Geometry: final body of the model. Coordinates: model frame, mm. A direction names the side the tool comes from. Give positions to 0.01 mm unless a question says otherwise; leave off trailing zeros. Loops run counter-clockwise (first coordinate to the right, second up) from the corner with the lowest first, then second, coordinate; pieces in that order, holes last. Notation, with made-up numbers: (-22.5, -3) - (19.5, -3) arc R19 cw to (19.5, 22) - close; hole circle Ø4 at (29, 15.25). An arc over 180 degrees is marked (long way). Answer in a Markdown table with one row per item.
from build123d import *

# Parameters (mm, degrees)
SKETCH1_W           = 37.338
SKETCH1_H           = 38.1
BOSS_EXTRUDE1_DEPTH = 63.5
SKETCH3_W           = 37.338
SKETCH3_H           = 10.16
CUT_EXTRUDE1_DEPTH  = 38.1
SKETCH4_W           = 37.338
SKETCH4_H           = 17.145
CUT_EXTRUDE2_DEPTH  = 19.05
SKETCH5_W           = 33.782
SKETCH5_H           = 10.16
CUT_EXTRUDE3_DEPTH  = 47.508537507
SKETCH6_W           = 2.54
SKETCH6_H           = 38.1
SKETCH6_W_2         = 1.778
CUT_EXTRUDE4_DEPTH  = 31.75


with BuildPart() as part:
    # Sketch1 → Boss-Extrude1 (new body)
    with BuildSketch(Plane(origin=(0, 0, 0), x_dir=(1, 0, 0), z_dir=(0, 1, 0))):
        Rectangle(SKETCH1_W, SKETCH1_H)
    extrude(amount=BOSS_EXTRUDE1_DEPTH)

    # Sketch3 → Cut-Extrude1 (cut)
    with BuildSketch(Plane(origin=(0, 63.5, 0), x_dir=(1, 0, 0), z_dir=(0, 1, 0))):
        Rectangle(SKETCH3_W, SKETCH3_H)
    extrude(amount=-CUT_EXTRUDE1_DEPTH, mode=Mode.SUBTRACT)

    # Sketch4 → Cut-Extrude2 (cut)
    with BuildSketch(Plane.XZ):
        Rectangle(SKETCH4_W, SKETCH4_H)
    extrude(amount=-CUT_EXTRUDE2_DEPTH, mode=Mode.SUBTRACT)

    # Sketch5 → Cut-Extrude3 (cut, through all)
    with BuildSketch(Plane(origin=(0, 25.4, 0), x_dir=(1, 0, 0), z_dir=(0, 1, 0))):
        Rectangle(SKETCH5_W, SKETCH5_H)
    extrude(amount=-CUT_EXTRUDE3_DEPTH, mode=Mode.SUBTRACT)

    # Sketch6 → Cut-Extrude4 (cut)
    with BuildSketch(Plane(origin=(0, 63.5, 0), x_dir=(1, 0, 0), z_dir=(0, 1, 0))):
        with Locations((17.399, 0)):
            Rectangle(SKETCH6_W, SKETCH6_H)
        with Locations((-17.78, 0)):
            Rectangle(SKETCH6_W_2, SKETCH6_H)
    extrude(amount=-CUT_EXTRUDE4_DEPTH, mode=Mode.SUBTRACT)


solid = part.part
Q1. Cut plane A-A (z = -1.5). Output: boundary loops of the cut face in (x, y), and give its area (3 significant figures).
Check values:
| item | result |
|---|---|
| outline | (-18.67, 19.05) - (-16.89, 19.05) - (-16.89, 25.4) - (-18.67, 25.4) - close; (16.89, 19.05) - (18.67, 19.05) - (18.67, 25.4) - (16.89, 25.4) - close |
| area | 22.6 mm² |
Q2. Material intervals for line 1 along Z through (x, y) = (5.5, 7.5); line 2 along Z through (x, y) = (-3.5, 43.5); line 3 along X through (y, z) = (52.5, 15), sorted ascending.
Check values:
| item | result |
|---|---|
| line 1 | -19.05 to -8.57, 8.57 to 19.05 |
| line 2 | -19.05 to -5.08, 5.08 to 19.05 |
| line 3 | -16.89 to 16.13 |
Q3. Cut plane D-D (z = 14). Output: boundary loops of the cut face in (x, y), and give its area (3 significant figures).
Check values:
| item | result |
|---|---|
| outline | (-18.67, 0) - (18.67, 0) - (18.67, 31.75) - (16.13, 31.75) - (16.13, 63.5) - (-16.89, 63.5) - (-16.89, 31.75) - (-18.67, 31.75) - close |
| area | 2,230 mm² |
Q4. Draft query along X for faces 1 (the flat face through (0, 42, -5.08)), 2 (the flat face through (18.669, 23, 0)), 3 (the flat face through (0, 9, -8.572)). Return one class per face: pulls with the +X half, pulls with the -X half, needs draft (parallel to the pull), parting line crosses it, or undercut.
Check values:
| item | result |
|---|---|
| face 1 | undercut |
| face 2 | pulls with the +X half |
| face 3 | needs draft |
Q5. Cut plane B-B (x = 13). Output: boundary loops of the cut face in (y, z), and give its area (3 significant figures).
Check values:
| item | result |
|---|---|
| outline | (0, -19.05) - (63.5, -19.05) - (63.5, -5.08) - (19.05, -5.08) - (19.05, -8.57) - (0, -8.57) - close; (0, 8.57) - (19.05, 8.57) - (19.05, 5.08) - (63.5, 5.08) - (63.5, 19.05) - (0, 19.05) - close |
| area | 1,640 mm² |
Q6. First-contact query: pin 1 (0.5 mm diameter, centred on x = -17.5, z = -14, fed in from +Y); pin 2 (0.5 mm diameter, centred on x = 17.5, z = 0, fed in from +Y); pin 3 (1 mm diameter, centred on x = -13.5, z = -13, fed in from -Y); pin 4 (13.5 mm diameter, centred on x = 4, z = 1.5, fed in from -Y). Flat tips, straight axial feed; report the tip coordinate or a pass-through.
Check values:
| item | result |
|---|---|
| pin 1 | y = 31.75 |
| pin 2 | y = 25.4 |
| pin 3 | y = 0 |
| pin 4 | y = 19.05 |
Q7. Cut plane C-C (y = 45.5). Output: boundary loops of the cut face in (x, z), and give its area (3 significant figures).
Check values:
| item | result |
|---|---|
| outline | (-16.89, -19.05) - (16.13, -19.05) - (16.13, -5.08) - (-16.89, -5.08) - close; (-16.89, 5.08) - (16.13, 5.08) - (16.13, 19.05) - (-16.89, 19.05) - close |
| area | 923 mm² |
Q8. Reachability of faces 4 (the flat face through (17, 31.75, -12)), 5 (the flat face through (0, 19.05, 6)), 6 (the flat face through (-18, 25.4, 0)), 7 (the flat face through (-16.891, 48, 12)) from +Z, -Z, +X, -X, +Y, -Y: full face, straight path, thin tool, end or side. Return the list, or none.
Check values:
| item | result |
|---|---|
| face 4 | +Z, -Z, +X, +Y |
| face 5 | +X, -X, -Y |
| face 6 | +X, -X, +Y |
| face 7 | +Z, -Z, -X, +Y |
